The model under review builds one solid part; all positions refer to its coordinate system, in mm. Face numbers are marked on the shaded views. A direction names the side the tool comes from. Coordinates: 2 decimals unless noted, no trailing zeros. Loops run counter-clockwise (first coordinate to the right, second up) from the corner with the lowest first, then second, coordinate; pieces in that order, holes last. Notation, with made-up numbers: (68, -20) - (121, -20) arc R26 ccw to (121, 7) - close; hole circle Ø8 at (42.25, -7.75). An arc over 180 degrees is marked (long way). Use a Markdown table: item, result. Add a question column.
1) For the marked faces 4 and 5, list the 3-axis set-ups (+Z, -Z, +X, -X, +Y, -Y) from which the entire face can be reached by the end or side of a thin tool; tool diameter is ignored.
2) Add section C-C, the plane x = 10. Give the boundary of the cut face in (y, z), and give its area (3 significant figures).
3) Add section A-A, the plane y = 60. Give the boundary of the cut face in (x, z).
4) To check wall thickness, follow L1, parallel to X at y = 59.15, z = -10; L2, parallel to Y at x = -8, z = -1.5; L3, parallel to Y at x = 7.75, z = 12. State the ranges of each line that lie inside material, in increasing order. Write a range as [from, to].
5) Add section D-D, the plane z = -10. Give the boundary of the cut face in (x, y).
6) The part is to be moulded in two halves that separate along X. For the marked faces 1, 2 and 3, say which applies: pulls with the +X half, pulls with the -X half, needs draft (parallel to the pull), parting line crosses it, or undercut.
7) Add section B-B, the plane z = 0. Give the boundary of the cut face in (x, y).
8) Clearance check with flat-ended pins moving along their axes: pin 1 (5 mm diameter, centred on x = -3.5, z = -7.5, fed in from -Y); pin 2 (5 mm diameter, centred on x = -10, z = -10, fed in from -Y); pin 3 (10 mm diameter, centred on x = 9.5, y = 30, fed in from +Z); pin 4 (8 mm diameter, centred on x = -10.5, y = 16, fed in from -Z). State where each tip first meets the part, or that it passes through.
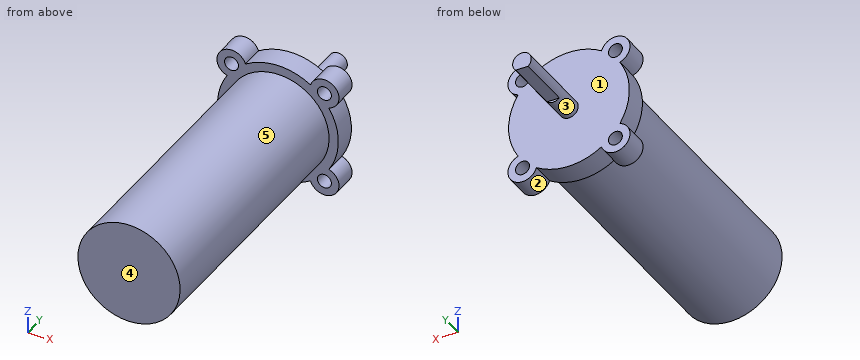
```python
from build123d import *

# Parameters (mm, degrees)
SKETCH1_R      = 11
EXTRUDE1_DEPTH = 62
SKETCH2_R      = 2
EXTRUDE2_DEPTH = 18
SKETCH3_R      = 1.5
SKETCH3_R_2    = 11
EXTRUDE3_DEPTH = 62
SKETCH4_R      = 20.921238725
SKETCH4_R_2    = 11
EXTRUDE4_DEPTH = 57
EXTRUDE5_START = -12
EXTRUDE5_DEPTH = 12


with BuildPart() as part:
    # Sketch1 → Extrude1 (new body)
    with BuildSketch(Plane(origin=(0, 0, 0), x_dir=(1, 0, 0), z_dir=(0, 1, 0))):
        with Locations(Location((0, 0, 0), (0, 0, 270))):
            Circle(SKETCH1_R)
    extrude(amount=EXTRUDE1_DEPTH)

    # Sketch2 → Extrude2 (add)
    with BuildSketch(Plane(origin=(0, 62, 0), x_dir=(1, 0, 0), z_dir=(0, 1, 0))):
        with Locations(Location((0, 0, 0), (0, 0, 270))):
            Circle(SKETCH2_R)
    extrude(amount=EXTRUDE2_DEPTH)

    # Sketch3 → Extrude3 (add)
    with BuildSketch(Plane.XZ):
        with BuildLine():
            ThreePointArc((10.951086395, -7.005262792), (13, 0), (10.951086395, 7.005262792))
            ThreePointArc((10.951086395, 7.005262792), (12.221825407, 12.221825407), (7.005262792, 10.951086395))
            ThreePointArc((7.005262792, 10.951086395), (0, 13), (-7.005262792, 10.951086395))
            ThreePointArc((-7.005262792, 10.951086395), (-12.221825407, 12.221825407), (-10.951086395, 7.005262792))
            ThreePointArc((-10.951086395, 7.005262792), (-13, 0), (-10.951086395, -7.005262792))
            ThreePointArc((-10.951086395, -7.005262792), (-12.221825407, -12.221825407), (-7.005262792, -10.951086395))
            ThreePointArc((-7.005262792, -10.951086395), (0, -13), (7.005262792, -10.951086395))
            ThreePointArc((7.005262792, -10.951086395), (12.221825407, -12.221825407), (10.951086395, -7.005262792))
        make_face()
        with Locations(Location((10, -10, 0), (0, 0, 270))):
            Circle(SKETCH3_R, mode=Mode.SUBTRACT)
        with Locations(Location((10, 10, 0), (0, 0, 270))):
            Circle(SKETCH3_R, mode=Mode.SUBTRACT)
        with Locations(Location((-10, 10, 0), (0, 0, 270))):
            Circle(SKETCH3_R, mode=Mode.SUBTRACT)
        with Locations(Location((-10, -10, 0), (0, 0, 270))):
            Circle(SKETCH3_R, mode=Mode.SUBTRACT)
        Circle(SKETCH3_R_2, mode=Mode.SUBTRACT)
    extrude(amount=-EXTRUDE3_DEPTH)

    # Sketch4 → Extrude4 (cut)
    with BuildSketch(Plane.XZ):
        Circle(SKETCH4_R)
        with Locations(Location((0, 0, 0), (0, 0, 270))):
            Circle(SKETCH4_R_2, mode=Mode.SUBTRACT)
    extrude(amount=-EXTRUDE4_DEPTH, mode=Mode.SUBTRACT)

    # Sketch5 → Extrude5 (cut)
    with BuildSketch(Plane(origin=(0, 80, 0), x_dir=(1, 0, 0), z_dir=(0, 1, 0)).offset(EXTRUDE5_START)):
        with BuildLine():
            Line((-1.322875656, 1.5), (1.322875656, 1.5))
            ThreePointArc((1.322875656, 1.5), (0, 2), (-1.322875656, 1.5))
        make_face()
    extrude(amount=EXTRUDE5_DEPTH, mode=Mode.SUBTRACT)


solid = part.part
```
From the geometry:
| question | item | result |
|---|---|---|
| 1 | face 4 | +Z, -Z, +X, -X, -Y |
| 1 | face 5 | -Y |
| 2 | outline | (0, -4.58) - (57, -4.58) - (57, -8.5) - (62, -8.5) - (62, 8.5) - (57, 8.5) - (57, 4.58) - (0, 4.58) - close; (57, -13.14) - (62, -13.14) - (62, -11.5) - (57, -11.5) - close; (57, 11.5) - (62, 11.5) - (62, 13.14) - (57, 13.14) - close |
| 2 | area | 624 mm^2 |
| 3 | outline | (-10.95, -7.01) arc R3.14 ccw (long way) to (-7.01, -10.95) arc R13 ccw to (7.01, -10.95) arc R3.14 ccw (long way) to (10.95, -7.01) arc R13 ccw to (10.95, 7.01) arc R3.14 ccw (long way) to (7.01, 10.95) arc R13 ccw to (-7.01, 10.95) arc R3.14 ccw (long way) to (-10.95, 7.01) arc R13 ccw to start; hole circle Ø3 at (-10, -10); hole circle Ø3 at (-10, 10); hole circle Ø3 at (10, -10); hole circle Ø3 at (10, 10) |
| 4 | L1 | x = [-13.14, -11.5], [-8.5, 8.5], [11.5, 13.14] |
| 4 | L2 | y = [0, 62] |
| 4 | L3 | y = [57, 62] |
| 5 | outline | (-13.14, 57) - (-11.5, 57) - (-11.5, 62) - (-13.14, 62) - close; (-8.5, 57) - (-4.58, 57) - (-4.58, 0) - (4.58, 0) - (4.58, 57) - (8.5, 57) - (8.5, 62) - (-8.5, 62) - close; (11.5, 57) - (13.14, 57) - (13.14, 62) - (11.5, 62) - close |
| 6 | face 1 | needs draft |
| 6 | face 2 | undercut |
| 6 | face 3 | parting line crosses it |
| 7 | outline | (-13, 57) - (-11, 57) - (-11, 0) - (11, 0) - (11, 57) - (13, 57) - (13, 62) - (2, 62) - (2, 80) - (-2, 80) - (-2, 62) - (-13, 62) - close |
| 8 | pin 1 | stops at y = 0 |
| 8 | pin 2 | stops at y = 57 |
| 8 | pin 3 | stops at z = 10.04 |
| 8 | pin 4 | stops at z = -8.87 |
